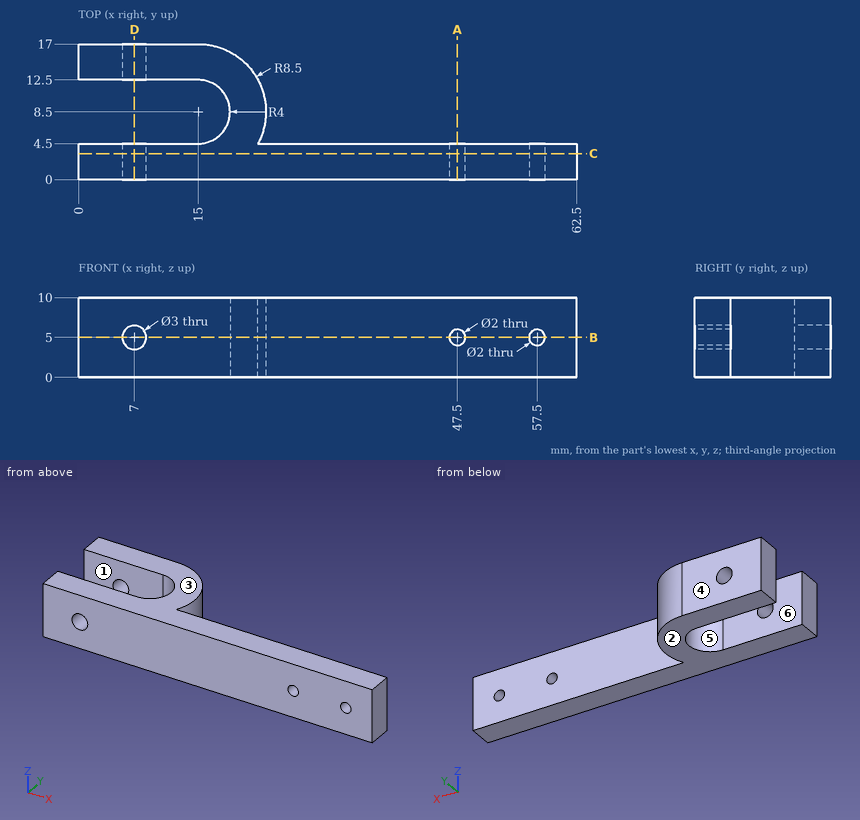
Part print with two shaded views. Sizes in mm from the minimum x, y, z corner. A direction names the side the tool comes from. Round coordinates to 2 decimals unless told otherwise and drop trailing zeros. Order: outer loops, then holes, each group sorted by start corner. A loop starts at its lowest first (then second) coordinate and runs counter-clockwise, first axis right, second up. Notation, with made-up numbers: (-26.75, 31.5) - (28.25, 31.5) arc R12 ccw to (28.25, 41.5) - close; hole circle Ø1 at (-21.75, -15.75). An arc over 180 degrees is marked (long way). Answer in a Markdown table with one row per item. Add a question column.
(1) Band-saw the part on C-C on y = 3.25. List the corners of the cut face in (x, z), and give its area (3 significant figures).
(2) Band-saw the part on B-B on z = 5. List the corners of the cut face in (x, y).
(3) Probe L1, parallel to Y at x = 6, z = 1.5; L2, parallel to Z at x = 47.5, y = 3.2; L3, parallel to Y at x = 50.5, z = 6.5. List the from-to ranges inside material, lowest first. Write a range as [from, to].
(4) Band-saw the part on D-D on x = 7. List the corners of the cut face in (y, z), and give its area (3 significant figures).
(5) Drop flat-ended pins along their axis: pin 1 Ø1 at (y, z) = (9.5, 4) entering from -X; pin 2 Ø3 at (x, z) = (6.5, 5) entering from +Y; pin 3 Ø2 at (x, z) = (40, 9) entering from +Y; pin 4 Ø5 at (x, z) = (24.5, 2.5) entering from +Y. Give the stop position or say it passes through.
(6) Mould opens along Y. For the marked faces 3, 4, 5 and 6 say: +Y half, -Y half, draft (parallel to the pull), parting line (faces both ways), or undercut.
(7) Band-saw the part on A-A on x = 47.5. List the corners of the cut face in (y, z).
(8) 3-axis set-ups, long thin cutter, end or side, ignore diameter. For the marked faces 1 and 2: which of +Z, -Z, +X, -X, +Y, -Y reach the whole face in a straight line?
Data:
| question | item | result |
|---|---|---|
| 1 | outline | (0, 0) - (62.5, 0) - (62.5, 10) - (0, 10) - close; hole circle Ø3 at (7, 5); hole circle Ø2 at (47.5, 5); hole circle Ø2 at (57.5, 5) |
| 1 | area | 612 mm^2 |
| 2 | outline | (0, 0) - (5.5, 0) - (5.5, 4.5) - (0, 4.5) - close; (0, 12.5) - (5.5, 12.5) - (5.5, 17) - (0, 17) - close; (8.5, 0) - (46.5, 0) - (46.5, 4.5) - (22.5, 4.5) arc R8.5 ccw to (15, 17) - (8.5, 17) - (8.5, 12.5) - (15, 12.5) arc R4 cw to (15, 4.5) - (8.5, 4.5) - close; (48.5, 0) - (56.5, 0) - (56.5, 4.5) - (48.5, 4.5) - close; (58.5, 0) - (62.5, 0) - (62.5, 4.5) - (58.5, 4.5) - close |
| 3 | L1 | y = [0, 4.5], [12.5, 17] |
| 3 | L2 | z = [0, 4], [6, 10] |
| 3 | L3 | y = [0, 4.5] |
| 4 | outline | (0, 0) - (4.5, 0) - (4.5, 3.5) - (0, 3.5) - close; (0, 6.5) - (4.5, 6.5) - (4.5, 10) - (0, 10) - close; (12.5, 0) - (17, 0) - (17, 3.5) - (12.5, 3.5) - close; (12.5, 6.5) - (17, 6.5) - (17, 10) - (12.5, 10) - close |
| 4 | area | 63.0 mm^2 |
| 5 | pin 1 | stops at x = 18.71 |
| 5 | pin 2 | stops at y = 17 |
| 5 | pin 3 | stops at y = 4.5 |
| 5 | pin 4 | stops at y = 13.32 |
| 6 | face 3 | draft |
| 6 | face 4 | +Y half |
| 6 | face 5 | undercut |
| 6 | face 6 | undercut |
| 7 | outline | (0, 0) - (4.5, 0) - (4.5, 4) - (0, 4) - close; (0, 6) - (4.5, 6) - (4.5, 10) - (0, 10) - close |
| 8 | face 1 | +Z, -Z, -X |
| 8 | face 2 | -Z, +X, -X, +Y, -Y |
